from build123d import *
from OCP.BRepAlgoAPI import BRepAlgoAPI_Cut
from OCP.TopTools import TopTools_ListOfShape
from OCP.BRepFilletAPI import BRepFilletAPI_MakeFillet

# Parameters (mm, degrees)
CROQUIS1_W              = 40
CROQUIS1_H              = 49.15
SALIENTE_EXTRUIR1_DEPTH = 5
CROQUIS5_W              = 6
CROQUIS5_H              = 4.995078359
CROQUIS5_H_2            = 5
CORTAR_EXTRUIR4_DEPTH   = 5
CROQUIS9_R              = 1.2
CORTAR_EXTRUIR8_DEPTH   = 32
REDONDEO1_R             = 2.5
CROQUIS12_W             = 39.999999512
CROQUIS12_H             = 44.15
CORTAR_EXTRUIR10_DEPTH  = 2.5
CROQUIS15_W             = 6
CROQUIS15_H             = 2.537629209
CORTAR_EXTRUIR11_DEPTH  = 0.01
CROQUIS17_W             = 2.5
CROQUIS17_H             = 4.997458943
SALIENTE_EXTRUIR2_DEPTH = 40
REDONDEO3_R             = 2.45
CROQUIS22_W             = 14
CROQUIS22_H             = 5
CORTAR_EXTRUIR13_DEPTH  = 5
CROQUIS25_W             = 5
CROQUIS25_H             = 7.03748993
CORTAR_EXTRUIR15_DEPTH  = 8
CROQUIS26_W             = 5
CROQUIS26_H             = 7
CORTAR_EXTRUIR16_DEPTH  = 8
CROQUIS29_W             = 5
CROQUIS29_H             = 4.997458943
SALIENTE_EXTRUIR3_DEPTH = 24
CROQUIS30_R             = 1.35
CORTAR_EXTRUIR17_DEPTH  = 24
REDONDEO4_R             = 2.5
REDONDEO4_R_2           = 2.4
CROQUIS31_W             = 2.5
CROQUIS31_H             = 4.997458943
CORTAR_EXTRUIR18_DEPTH  = 24
CROQUIS32_W             = 8.001194755
CROQUIS32_H             = 7
CORTAR_EXTRUIR19_DEPTH  = 2.5
CROQUIS33_W             = 8.001407562
CROQUIS33_H             = 6.993550445
CORTAR_EXTRUIR20_DEPTH  = 2.5
CROQUIS36_R             = 1.35
SALIENTE_EXTRUIR4_DEPTH = 3
SALIENTE_EXTRUIR5_START = 3
CROQUIS37_R             = 1.35
SALIENTE_EXTRUIR5_DEPTH = 3
REDONDEO5_R             = 2.45
REDONDEO6_R             = 2.45


# Some blends are built 0.0001 mm under size
with BuildPart() as part:
    # Croquis1 → Saliente-Extruir1 (new body)
    with BuildSketch(Plane.XY):
        Rectangle(CROQUIS1_W, CROQUIS1_H)
    extrude(amount=SALIENTE_EXTRUIR1_DEPTH)

    # Croquis5 → Cortar-Extruir4 (cut)
    with BuildSketch(Plane.XY):
        with Locations((-17, 22.077460821)):
            Rectangle(CROQUIS5_W, CROQUIS5_H)
        with Locations((17, 22.075)):
            Rectangle(CROQUIS5_W, CROQUIS5_H_2)
    extrude(amount=CORTAR_EXTRUIR4_DEPTH, mode=Mode.SUBTRACT)

    # Croquis9 → Cortar-Extruir8 (cut)
    with BuildSketch(Plane.ZY.offset(14)):
        with Locations((2.5, 22.075)):
            Circle(CROQUIS9_R)
    extrude(amount=-CORTAR_EXTRUIR8_DEPTH, mode=Mode.SUBTRACT)

    # Redondeo1
    redondeo1_edges = [part.edges().sort_by_distance(p)[0] for p in [
        (0, 24.575, 5),
        (0, 24.575, 0),
    ]]
    fillet(redondeo1_edges, radius=REDONDEO1_R - 0.0001)  # a hair under: the kernel refuses the full size


with BuildPart() as cortar_extruir10_tool:
    # Croquis12 → Cortar-Extruir10 (new body)
    with BuildSketch(Plane.XY.offset(5)):
        with Locations((2.44e-07, -2.5)):
            Rectangle(CROQUIS12_W, CROQUIS12_H)
    extrude(amount=-CORTAR_EXTRUIR10_DEPTH)


with BuildPart() as part_1:
    add(part.part)

    # Cortar-Extruir10: cut by cortar_extruir10_tool, with a tolerance
    cortar_extruir10_stock = TopTools_ListOfShape()
    cortar_extruir10_stock.Append(part_1.part.wrapped)
    cortar_extruir10_tools = TopTools_ListOfShape()
    cortar_extruir10_tools.Append(cortar_extruir10_tool.part.wrapped)
    cortar_extruir10_cut = BRepAlgoAPI_Cut()
    cortar_extruir10_cut.SetArguments(cortar_extruir10_stock)
    cortar_extruir10_cut.SetTools(cortar_extruir10_tools)
    cortar_extruir10_cut.SetFuzzyValue(0.00001)
    cortar_extruir10_cut.Build()
    add(Compound.cast(cortar_extruir10_cut.Shape()).solids(), mode=Mode.REPLACE)

    # Croquis15 → Cortar-Extruir11 (cut)
    with BuildSketch(Plane(origin=(0, 19.579921641, 0), x_dir=(1, 0, 0), z_dir=(0, 1, 0))):
        with Locations((-17, -3.768814605)):
            Rectangle(CROQUIS15_W, CROQUIS15_H)
    extrude(amount=-CORTAR_EXTRUIR11_DEPTH, mode=Mode.SUBTRACT)

    # Croquis17 → Saliente-Extruir2 (add)
    with BuildSketch(Plane.ZY.offset(20)):
        with Locations((-1.25, -14.076270529)):
            Rectangle(CROQUIS17_W, CROQUIS17_H)
    extrude(amount=-SALIENTE_EXTRUIR2_DEPTH)

    # Redondeo3
    redondeo3_edges = [part_1.edges().sort_by_distance(p)[0] for p in [
        (0, -16.575, -2.5),
        (0, -11.577541057, -2.5),
    ]]
    fillet(redondeo3_edges, radius=REDONDEO3_R)

    # Croquis22 → Cortar-Extruir13 (cut)
    with BuildSketch(Plane.XZ.offset(16.575)):
        with Locations((0, -2.5)):
            Rectangle(CROQUIS22_W, CROQUIS22_H)
    extrude(amount=-CORTAR_EXTRUIR13_DEPTH, mode=Mode.SUBTRACT)

    # Croquis25 → Cortar-Extruir15 (cut)
    with BuildSketch(Plane(origin=(20, 0, 0), x_dir=(0, 0, -1), z_dir=(1, 0, 0))):
        with Locations((0, -14.06270459)):
            Rectangle(CROQUIS25_W, CROQUIS25_H)
    extrude(amount=-CORTAR_EXTRUIR15_DEPTH, mode=Mode.SUBTRACT)

    # Croquis26 → Cortar-Extruir16 (cut)
    with BuildSketch(Plane.ZY.offset(20)):
        with Locations((0, -14.075)):
            Rectangle(CROQUIS26_W, CROQUIS26_H)
    extrude(amount=-CORTAR_EXTRUIR16_DEPTH, mode=Mode.SUBTRACT)

    # Croquis29 → Saliente-Extruir3 (add)
    with BuildSketch(Plane(origin=(12, 0, 0), x_dir=(0, 0, -1), z_dir=(1, 0, 0))):
        with Locations((-2.5, -14.076270529)):
            Rectangle(CROQUIS29_W, CROQUIS29_H)
    extrude(amount=-SALIENTE_EXTRUIR3_DEPTH)

    # Croquis30 → Cortar-Extruir17 (cut)
    with BuildSketch(Plane.ZY.offset(12)):
        with Locations((2.5, -14.076270528)):
            Circle(CROQUIS30_R)
    extrude(amount=-CORTAR_EXTRUIR17_DEPTH, mode=Mode.SUBTRACT)

    # Redondeo4
    redondeo4_edges_1 = [part_1.edges().sort_by_distance(p)[0] for p in [
        (0, -16.575, 5),
    ]]
    redondeo4_edges_2 = [part_1.edges().sort_by_distance(p)[0] for p in [
        (0, -11.577541057, 5),
    ]]
    redondeo4 = BRepFilletAPI_MakeFillet(part_1.part.solid().wrapped)
    for e in redondeo4_edges_1:
        redondeo4.Add(REDONDEO4_R - 0.0001, e.wrapped)
    for e in redondeo4_edges_2:
        redondeo4.Add(REDONDEO4_R_2 - 0.0001, e.wrapped)
    add(Compound.cast(redondeo4.Shape()), mode=Mode.REPLACE)  # a hair under: the kernel refuses the full size

    # Croquis31 → Cortar-Extruir18 (cut)
    with BuildSketch(Plane(origin=(12, 0, 0), x_dir=(0, 0, -1), z_dir=(1, 0, 0))):
        with Locations((1.25, -14.076270529)):
            Rectangle(CROQUIS31_W, CROQUIS31_H)
    extrude(amount=-CORTAR_EXTRUIR18_DEPTH, mode=Mode.SUBTRACT)

    # Croquis32 → Cortar-Extruir19 (cut)
    with BuildSketch(Plane.XY.offset(2.5)):
        with Locations((-16.000597378, -21.075)):
            Rectangle(CROQUIS32_W, CROQUIS32_H)
    extrude(amount=-CORTAR_EXTRUIR19_DEPTH, mode=Mode.SUBTRACT)

    # Croquis33 → Cortar-Extruir20 (cut)
    with BuildSketch(Plane.XY.offset(2.5)):
        with Locations((16.000703781, -21.078224778)):
            Rectangle(CROQUIS33_W, CROQUIS33_H)
    extrude(amount=-CORTAR_EXTRUIR20_DEPTH, mode=Mode.SUBTRACT)

    # Croquis36 → Saliente-Extruir4 (add)
    with BuildSketch(Plane(origin=(12, 0, 0), x_dir=(0, 0, -1), z_dir=(1, 0, 0))):
        Polygon((0, -24.575), (-2.5, -24.575), (-2.5, -16.575), (-5, -16.575), (-5, -11.576082189), (-2.5, -11.577541057), (-2.5, -10.543959625), (0, -10.543959625), align=None)
        with Locations(Location((-2.5, -14.076270528, 0), (0, 0, 180))):
            Circle(CROQUIS36_R, mode=Mode.SUBTRACT)
    extrude(amount=SALIENTE_EXTRUIR4_DEPTH)

    # Croquis37 → Saliente-Extruir5 (add)
    with BuildSketch(Plane.ZY.offset(12).offset(SALIENTE_EXTRUIR5_START)):
        Polygon((0, -24.575), (2.5, -24.575), (2.5, -16.575), (5, -16.575), (5, -11.57700903), (2.5, -11.577541057), (2.5, -10.575), (0, -10.575), align=None)
        with Locations((2.5, -14.076270528)):
            Circle(CROQUIS37_R, mode=Mode.SUBTRACT)
    extrude(amount=-SALIENTE_EXTRUIR5_DEPTH)

    # Redondeo5
    # the kernel refuses this fillet: 2.45 mm, written as the material it takes off along each edge
    with BuildSketch(Plane(origin=(-2.708580643, -11.576082189, 5), x_dir=(0, -1, 0), z_dir=(1, 0, 0))) as redondeo5_piece_1:
        with BuildLine():
            CenterArc((REDONDEO5_R * 1.00058371722, REDONDEO5_R), REDONDEO5_R, 179.966565226, 90.033434774)
            Line((REDONDEO5_R * 0.000583887478773, REDONDEO5_R * 1.00058354685), (-REDONDEO5_R * 0.019416109116, REDONDEO5_R * 1.00059521779))
            Line((-REDONDEO5_R * 0.019416109116, REDONDEO5_R * 1.00059521779), (-REDONDEO5_R * 0.0200116743443, -REDONDEO5_R * 0.02))
            Line((-REDONDEO5_R * 0.0200116743443, -REDONDEO5_R * 0.02), (REDONDEO5_R * 1.00058371722, -REDONDEO5_R * 0.02))
            Line((REDONDEO5_R * 1.00058371722, -REDONDEO5_R * 0.02), (REDONDEO5_R * 1.00058371722, 0))
        make_face()
    extrude(amount=32.417161286, mode=Mode.SUBTRACT)
    with BuildSketch(Plane(origin=(-2.7, -16.575, 5), x_dir=(0, 0, -1), z_dir=(1, 0, 0))) as redondeo5_piece_2:
        with BuildLine():
            CenterArc((REDONDEO5_R, REDONDEO5_R), REDONDEO5_R, 180, 90)
            Line((0, REDONDEO5_R), (-REDONDEO5_R * 0.02, REDONDEO5_R))
            Line((-REDONDEO5_R * 0.02, REDONDEO5_R), (-REDONDEO5_R * 0.02, -REDONDEO5_R * 0.02))
            Line((-REDONDEO5_R * 0.02, -REDONDEO5_R * 0.02), (REDONDEO5_R, -REDONDEO5_R * 0.02))
            Line((REDONDEO5_R, -REDONDEO5_R * 0.02), (REDONDEO5_R, 0))
        make_face()
    extrude(amount=32.4, mode=Mode.SUBTRACT)
    with BuildSketch(Plane(origin=(-29.703128651, -11.57700903, 5), x_dir=(0, -1, 0), z_dir=(1, 0, 0))) as redondeo5_piece_3:
        with BuildLine():
            CenterArc((REDONDEO5_R * 1.00021283342, REDONDEO5_R), REDONDEO5_R, 179.987806841, 90.012193159)
            Line((REDONDEO5_R * 0.000212856064231, REDONDEO5_R * 1.00021281077), (-REDONDEO5_R * 0.0197871434829, REDONDEO5_R * 1.00021706699))
            Line((-REDONDEO5_R * 0.0197871434829, REDONDEO5_R * 1.00021706699), (-REDONDEO5_R * 0.0200042566684, -REDONDEO5_R * 0.02))
            Line((-REDONDEO5_R * 0.0200042566684, -REDONDEO5_R * 0.02), (REDONDEO5_R * 1.00021283342, -REDONDEO5_R * 0.02))
            Line((REDONDEO5_R * 1.00021283342, -REDONDEO5_R * 0.02), (REDONDEO5_R * 1.00021283342, 0))
        make_face()
    extrude(amount=32.406257303, mode=Mode.SUBTRACT)

    # Redondeo6
    redondeo6_edges = [part_1.edges().sort_by_distance(p)[0] for p in [
        (-13.5, -16.575, 5),
    ]]
    fillet(redondeo6_edges, radius=REDONDEO6_R)


solid = part_1.part
Verification items for the finished model (mm, model axes). A direction names the side the tool comes from. Round coordinates to 2 decimals unless told otherwise and drop trailing zeros. Write each loop counter-clockwise with the first axis right and the second up, starting at its lowest first coordinate (ties: lowest second). Pieces come first, ordered by that corner, then holes.
(1) Section check B-B (z = 1.85). Enter the section's corners in (x, y) (3 decimals), plus the area to 3 significant figures.
Returned:
outline: (-20, -10.575) - (-15, -10.575) - (-15, -12.893) - (15, -12.893) - (15, -10.544) - (20, -10.544) - (20, 19.575) - (14, 19.575) - (14, 21.066) - (-14, 21.066) - (-14, 19.58) - (-20, 19.58) - close; (-15, -24.575) - (15, -24.575) - (15, -15.259) - (-15, -15.259) - close; (-14, 23.084) - (14, 23.084) - (14, 24.489) - (-14, 24.489) - close
area: 1,640 mm2
(2) Section check D-D (y = 18). Enter the section's corners in (x, z), plus the area to 3 significant figures.
Returned:
outline: (-20, 0) - (20, 0) - (20, 2.5) - (-20, 2.5) - close
area: 100 mm2
(3) Mould release check, pull along Y, two halves, no side actions. Record for faces 1 (the cylindrical face through (-6.272, -12.276, 4.263)), 2 (the flat face through (15, -17, 2)), 3 (the cylindrical face through (-13.48, -15.84, 4.3)): pulls with the +Y half, pulls with the -Y half, needs draft (parallel to the pull), parting line crosses it, or undercut.
Returned:
face 1: undercut
face 2: needs draft
face 3: pulls with the -Y half
(4) Section check A-A (x = 1). Give the number of separate pieces and of enclosed holes in the cut face, plus the area to 3 significant figures.
Returned:
separate pieces: 1
enclosed holes: 2
area: 132 mm2
(5) Material ranges on line 1 (Y direction, x = -9, z = 2.7) (3 decimals); line 2 (Z direction, x = 11.5, y = -9); line 3 (X direction, y = 21, z = 3.8), recorded low to high.
Returned:
line 1: y = -16.567 to -15.411, -12.741 to -11.582, 19.575 to 20.892, 23.258 to 24.567
line 2: z = 0 to 2.5
line 3: x = -14 to 14
(6) Access from +Z, -Z, +X, -X, +Y, -Y to the whole of each face (thin tool, end or side, straight path). Record for faces 4 (the flat face through (0, 19.575, 4)), 5 (the flat face through (0, -21, 2.5)), 6 (the flat face through (-18, -10.575, 1)), 7 (the flat face through (17, 19.575, 1)), 8 (the flat face through (-17, 19.58, 1)).
Returned:
face 4: +Z, +X, -X
face 5: +Z, +X, -X, -Y
face 6: +Z, -Z, -X, -Y
face 7: +Z, -Z, +X, +Y
face 8: +Z, -Z, -X, +Y
(7) Depth check by flat-ended pin: pin 1 Ø1.5 at (x, y) = (-8, -2) entering from +Z; pin 2 Ø1.3 at (x, z) = (-16.5, 1.5) entering from +Y; pin 3 Ø1.5 at (y, z) = (-18, 3) entering from -X. Enter the tip coordinate at first touch or a pass-through.
Returned:
pin 1: stops at z = 2.5
pin 2: stops at y = 19.58
pin 3: stops at x = -15
